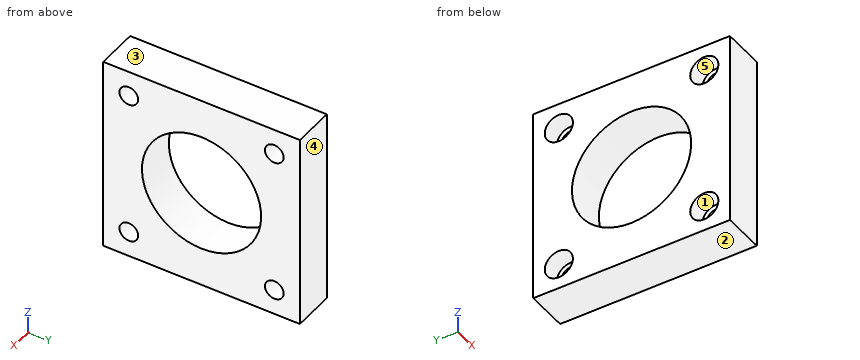
```python
from build123d import *

# Parameters (mm, degrees)
SKETCH37_W           = 41.91
SKETCH37_H           = 41.91
SKETCH37_R           = 2.999999969
SKETCH37_R_2         = 12.7
SKETCH37_R_3         = 2
BOSS_EXTRUDE27_DEPTH = 8.89
SKETCH37_9_R         = 2.999999969
CUT_EXTRUDE1_DEPTH   = 4.000000128


with BuildPart() as part:
    # Sketch37 → Boss-Extrude27 (new body)
    with BuildSketch(Plane(origin=(0, 0, 0), x_dir=(0, 0, -1), z_dir=(1, 0, 0))):
        Rectangle(SKETCH37_W, SKETCH37_H)
        with Locations((15.5, -15.5)):
            Circle(SKETCH37_R, mode=Mode.SUBTRACT)
        with Locations((-15.5, -15.5)):
            Circle(SKETCH37_R, mode=Mode.SUBTRACT)
        with Locations((-15.5, 15.5)):
            Circle(SKETCH37_R, mode=Mode.SUBTRACT)
        with Locations((15.5, 15.5)):
            Circle(SKETCH37_R, mode=Mode.SUBTRACT)
        Circle(SKETCH37_R_2, mode=Mode.SUBTRACT)
        with Locations((15.5, 15.5)):
            Circle(SKETCH37_R)
        with Locations((15.5, 15.5)):
            Circle(SKETCH37_R_3, mode=Mode.SUBTRACT)
        with Locations((-15.5, 15.5)):
            Circle(SKETCH37_R)
        with Locations((-15.5, 15.5)):
            Circle(SKETCH37_R_3, mode=Mode.SUBTRACT)
        with Locations((-15.5, -15.5)):
            Circle(SKETCH37_R)
        with Locations((-15.5, -15.5)):
            Circle(SKETCH37_R_3, mode=Mode.SUBTRACT)
        with Locations((15.5, -15.5)):
            Circle(SKETCH37_R)
        with Locations((15.5, -15.5)):
            Circle(SKETCH37_R_3, mode=Mode.SUBTRACT)
    extrude(amount=BOSS_EXTRUDE27_DEPTH)

    # Sketch37_9 → Cut-Extrude1 (cut)
    with BuildSketch(Plane(origin=(0, 0, 0), x_dir=(0, 0, -1), z_dir=(1, 0, 0))):
        with Locations((15.5, 15.5)):
            Circle(SKETCH37_9_R)
        with Locations((-15.5, 15.5)):
            Circle(SKETCH37_9_R)
        with Locations((-15.5, -15.5)):
            Circle(SKETCH37_9_R)
        with Locations((15.5, -15.5)):
            Circle(SKETCH37_9_R)
    extrude(amount=CUT_EXTRUDE1_DEPTH, mode=Mode.SUBTRACT)


solid = part.part
```
Verification items for the finished model (mm, model axes). Face numbers are marked on the shaded views. A direction names the side the tool comes from. Round coordinates to 2 decimals unless told otherwise and drop trailing zeros. Write each loop counter-clockwise with the first axis right and the second up, starting at its lowest first coordinate (ties: lowest second). Pieces come first, ordered by that corner, then holes.
1. Section check A-A on y = 0. Enter the section's corners in (x, z) (3 decimals), plus the area to 3 significant figures.
2. Access from +Z, -Z, +X, -X, +Y, -Y to the whole of each face (thin tool, end or side, straight path). Record for the marked faces 4 and 5.
3. Draft check along Z on the marked faces 1, 2 and 3. Enter one of: +Z half, -Z half, draft (parallel to the pull), parting line (faces both ways), or undercut.
4. Gauge pin test, flat ends, axial feed: P1, Ø5, axis at y = 15.5, z = -15.5, coming from the +X side; P2, Ø5.5, axis at y = -15.5, z = 15.5, coming from the -X side. Record the tip position at first contact, or that the pin passes through.
5. Section check C-C on y = 15.5. Enter the section's corners in (x, z) (3 decimals).
6. Scan lines: L1, parallel to Y at x = 2, z = -15.5 (3 decimals); L2, parallel to Y at x = 6.75, z = 15.5 (3 decimals). Record each from-to range of solid material in increasing order.
Answer:
1. outline: (0, -20.955) - (8.89, -20.955) - (8.89, -12.7) - (0, -12.7) - close; (0, 12.7) - (8.89, 12.7) - (8.89, 20.955) - (0, 20.955) - close
1. area: 147 mm2
2. face 4: +Z, -Z, +X, -X, +Y
2. face 5: -X
3. face 1: undercut
3. face 2: -Z half
3. face 3: +Z half
4. P1: stops at x = 8.89
4. P2: stops at x = 4
5. outline: (0, -20.955) - (8.89, -20.955) - (8.89, -17.5) - (4, -17.5) - (4, -18.5) - (0, -18.5) - close; (0, -12.5) - (4, -12.5) - (4, -13.5) - (8.89, -13.5) - (8.89, 13.5) - (4, 13.5) - (4, 12.5) - (0, 12.5) - close; (0, 18.5) - (4, 18.5) - (4, 17.5) - (8.89, 17.5) - (8.89, 20.955) - (0, 20.955) - close
6. L1: y = -20.955 to -18.5, -12.5 to 12.5, 18.5 to 20.955
6. L2: y = -20.955 to -17.5, -13.5 to 13.5, 17.5 to 20.955
